Study the drawing (mm; zero at the part's minimum x, y, z) and answer. A direction names the side the tool comes from. Round coordinates to 2 decimals unless told otherwise and drop trailing zeros. Write each loop counter-clockwise with the first axis right and the second up, starting at its lowest first coordinate (ties: lowest second). Pieces come first, ordered by that corner, then holes.
(1) A cutting plane is placed at C-C, the plane x = 11. Give the vertices of the cut face in (y, z) (1 decimal).
(2) For the marked faces 4, 5 and 6, determine the directions among +Z, -Z, +X, -X, +Y, -Y from which every point of the face is accessible in a straight line to the end or side of a thin tool.
(3) A cutting plane is placed at B-B, the plane z = 14. Give the vertices of the cut face in (x, y).
(4) Each of these flat-tipped pins is pushed along its axis until it touches: pin 1 Ø1.5 at (x, z) = (14, 13.5) entering from -Y; pin 2 Ø3 at (x, y) = (23, 11) entering from +Z; pin 3 Ø4 at (x, y) = (13.5, 11) entering from -Z; pin 4 Ø6 at (x, y) = (5, 7) entering from +Z (1 decimal). Where does it stop, or does it pass through?
(5) The mould has two halves that part along Z. Classify the marked faces 1, 2 and 3: +Z half, -Z half, draft (parallel to the pull), parting line (faces both ways), or undercut.
(6) A cutting plane is placed at D-D, the plane y = 6.25. Give the vertices of the cut face in (x, z) (1 decimal), and give its area (3 significant figures).
(7) A cutting plane is placed at A-A, the plane y = 2.5. Give the vertices of the cut face in (x, z) (1 decimal).
(8) Find the intervals of material crossed by probe 1 along Y at (x, z) = (3.5, 26); probe 2 along Z at (x, y) = (15.5, 10); probe 3 along Z at (x, y) = (11, 7.25) (1 decimal), in increasing order.
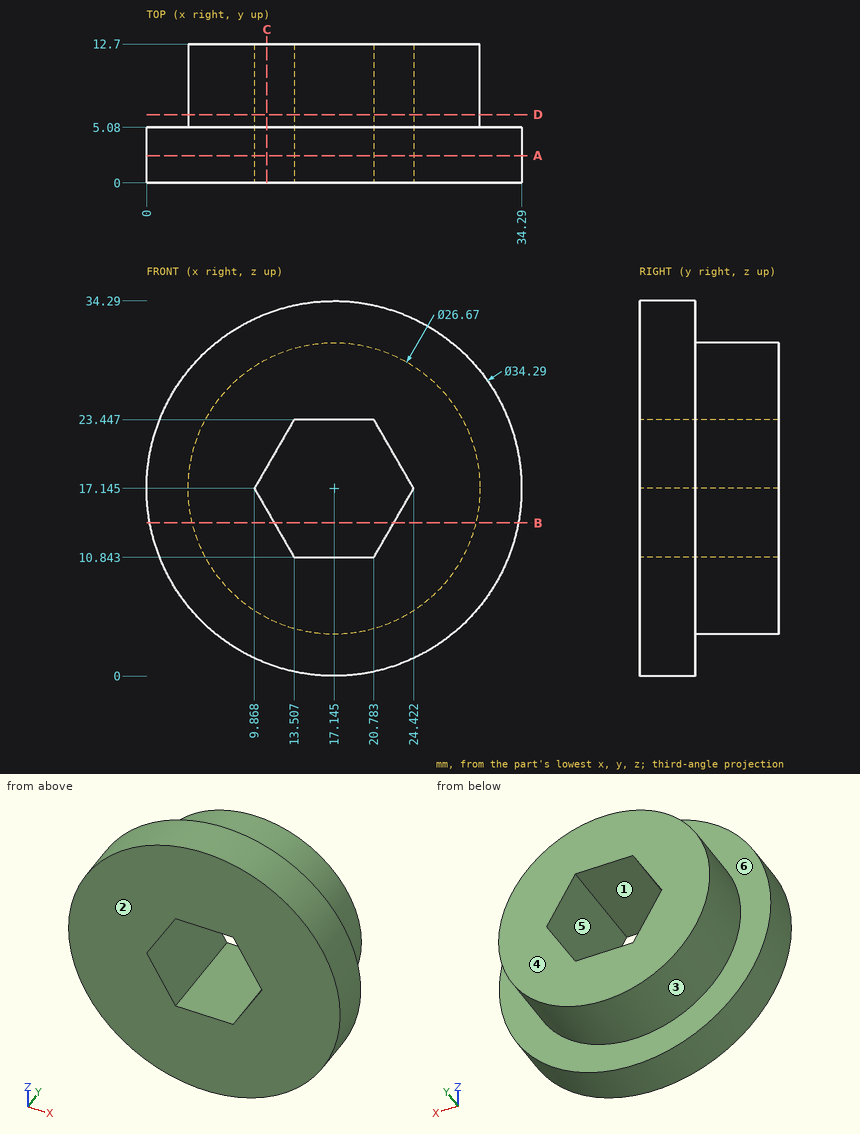
Solutions:
1. outline: (0, 1.1) - (5.1, 1.1) - (5.1, 5.3) - (12.7, 5.3) - (12.7, 15.2) - (0, 15.2) - close; (0, 19.1) - (12.7, 19.1) - (12.7, 29) - (5.1, 29) - (5.1, 33.2) - (0, 33.2) - close
2. face 4: +Z, -Z, +X, -X, +Y
2. face 5: +Y, -Y
2. face 6: +Y
3. outline: (0.29, 0) - (11.68, 0) - (11.68, 12.7) - (4.19, 12.7) - (4.19, 5.08) - (0.29, 5.08) - close; (22.61, 0) - (34, 0) - (34, 5.08) - (30.1, 5.08) - (30.1, 12.7) - (22.61, 12.7) - close
4. pin 1: passes through
4. pin 2: stops at z = 29.75
4. pin 3: stops at z = 3.91
4. pin 4: stops at z = 31.2
5. face 1: undercut
5. face 2: draft
5. face 3: parting line
6. outline: circle Ø26.7 at (17.1, 17.1); hole (9.9, 17.1) - (13.5, 10.8) - (20.8, 10.8) - (24.4, 17.1) - (20.8, 23.4) - (13.5, 23.4) - close
6. area: 421 mm2
7. outline: circle Ø34.3 at (17.1, 17.1); hole (9.9, 17.1) - (13.5, 10.8) - (20.8, 10.8) - (24.4, 17.1) - (20.8, 23.4) - (13.5, 23.4) - close
8. probe 1: y = 0 to 5.08
8. probe 2: z = 3.91 to 10.84, 23.45 to 30.38
8. probe 3: z = 5.3 to 15.2, 19.1 to 29
